Job drawing, mm, ordinate dimensions from the low corner. One solid piece. Round coordinates to 2 decimals unless told otherwise and drop trailing zeros. Loops run counter-clockwise (first coordinate to the right, second up) from the corner with the lowest first, then second, coordinate; pieces in that order, holes last. Notation, with made-up numbers: M -7,51.5 L 36,51.5 A8 ccw 36,66.5 Z; hole C 7,48 d5. An arc over 180 degrees is marked long. Write each question's results on one line, items separated by ' | '. Start each with the question number.
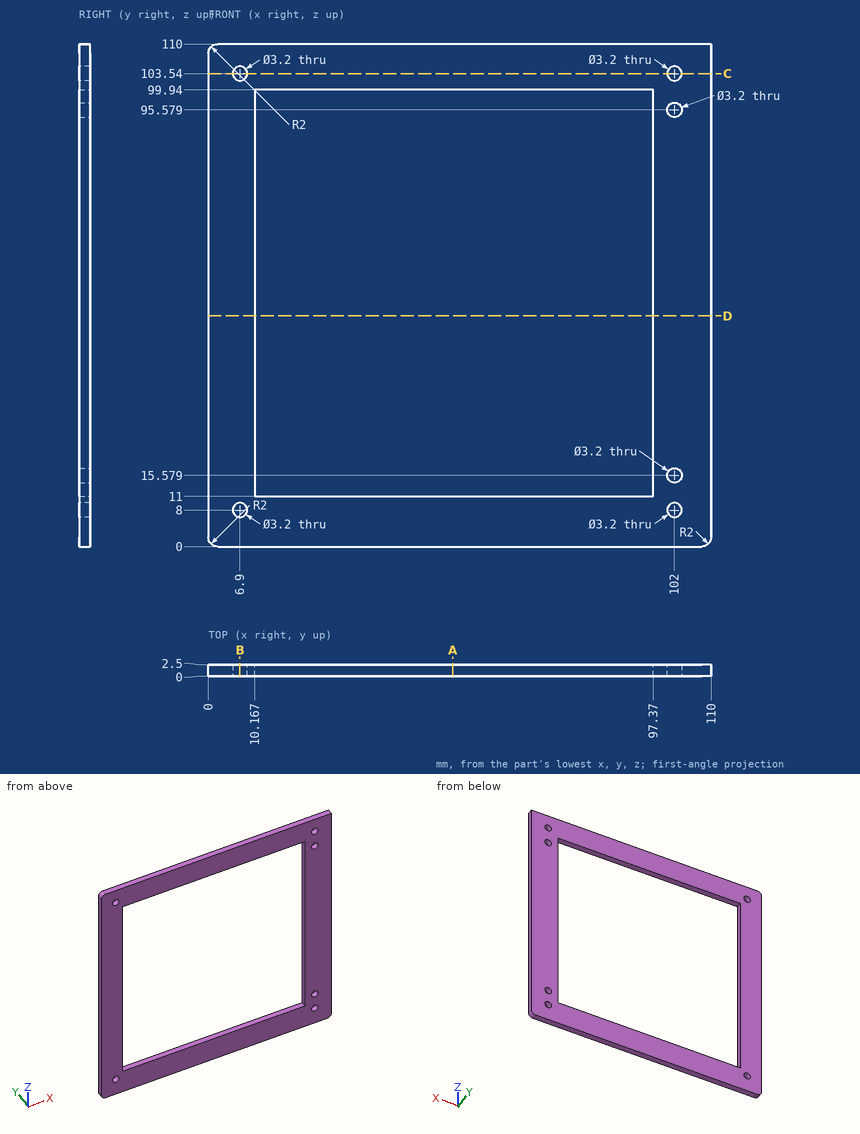
Item 1: Saw through at A-A, the plane x = 53.5. Give the cut face in (y, z).
Item 2: Drop a flat-ended pin along its axis: pin 1 (2 mm diameter, centred on x = 11.5, z = 73, fed in from +Y). Give the stop position or say it passes through.
Item 3: Saw through at D-D, the plane z = 50.5. Give the cut face in (x, y).
Item 4: Drill centre lines: line 1 along Z through (x, y) = (102, 1.95); line 2 along X through (y, z) = (2.45, 25.5); line 3 along Z through (x, y) = (48, 1.7). Where is each one in solid material? Low to high. Write a range as [from, to].
Item 5: Saw through at C-C, the plane z = 103.54. Give the cut face in (x, y), then the cut area to 3 significant figures.
Item 6: Saw through at B-B, the plane x = 6.9. Give the cut face in (y, z).
Working result:
1) outline: M 0,0 L 2.5,0 L 2.5,11 L 0,11 Z; M 0,99.94 L 2.5,99.94 L 2.5,110 L 0,110 Z
2) pin 1: passes through
3) outline: M 0,0 L 10.17,0 L 10.17,2.5 L 0,2.5 Z; M 97.37,0 L 110,0 L 110,2.5 L 97.37,2.5 Z
4) line 1: z = [0, 6.4], [9.6, 13.98], [17.18, 93.98], [97.18, 101.94], [105.14, 110] | line 2: x = [0, 10.17], [97.37, 110] | line 3: z = [0, 11], [99.94, 110]
5) outline: M 0,0 L 5.3,0 L 5.3,2.5 L 0,2.5 Z; M 8.5,0 L 100.4,0 L 100.4,2.5 L 8.5,2.5 Z; M 103.6,0 L 110,0 L 110,2.5 L 103.6,2.5 Z | area: 259 mm²
6) outline: M 0,0 L 2.5,0 L 2.5,6.4 L 0,6.4 Z; M 0,9.6 L 2.5,9.6 L 2.5,101.94 L 0,101.94 Z; M 0,105.14 L 2.5,105.14 L 2.5,110 L 0,110 Z
